Source: CAD feature listing. Evaluate the final solid. Frame: model axes, mm. Give positions to 0.01 mm unless a question says otherwise; leave off trailing zeros. Order: outer loops, then holes, each group sorted by start corner. A loop starts at its lowest first (then second) coordinate and runs counter-clockwise, first axis right, second up. Notation, with made-up numbers: M 9,-3 L 56,-3 A23 ccw 56,34 Z; hole C 45.25,24.25 d11. An arc over 180 degrees is marked long. Answer in a Markdown table with one row per item. Add a question column.
(1) Section query A-A, the plane y = 3.75. Return loops of the section in (x, z) (3 decimals).
(2) Section query B-B, the plane x = 0. Return loops of the section in (y, z) (3 decimals).
(3) Material intervals for line 1 along Z through (x, y) = (0, -11.05); line 2 along Y through (x, z) = (-5.5, 93) (3 decimals); line 3 along X through (y, z) = (10.7, 43.18), sorted ascending.
(4) Pin query (flat end, axial travel): P1, Ø20.5, axis at x = 0, z = 43.18, coming from the +Y side. Return the tip coordinate at first contact, or that it passes through.
(5) Section query C-C, the plane z = 43.18. Return loops of the section in (x, y) (3 decimals), plus the area to 3 significant figures.
(6) Section query D-D, the plane z = 349. Return loops of the section in (x, y) (3 decimals).
from build123d import *

# Parameters (mm, degrees)
SKETCH1_W           = 50.8
SKETCH1_H           = 25.4
SKETCH1_W_2         = 44.45
SKETCH1_H_2         = 19.05
EXTRUDE_THIN1_DEPTH = 508
SKETCH2_R           = 6.35
CUT_EXTRUDE1_DEPTH  = 26.4


with BuildPart() as part:
    # Sketch1 → Extrude-Thin1 (new body)
    with BuildSketch(Plane.XY):
        Rectangle(SKETCH1_W, SKETCH1_H)
        Rectangle(SKETCH1_W_2, SKETCH1_H_2, mode=Mode.SUBTRACT)
    extrude(amount=EXTRUDE_THIN1_DEPTH)

    # Sketch2 → Cut-Extrude1 (cut, through all)
    with BuildSketch(Plane(origin=(0, 12.7, 0), x_dir=(1, 0, 0), z_dir=(0, 1, 0))):
        with Locations((0, -464.82)):
            Circle(SKETCH2_R)
        with Locations((0, -43.18)):
            Circle(SKETCH2_R)
    extrude(amount=-CUT_EXTRUDE1_DEPTH, mode=Mode.SUBTRACT)


solid = part.part
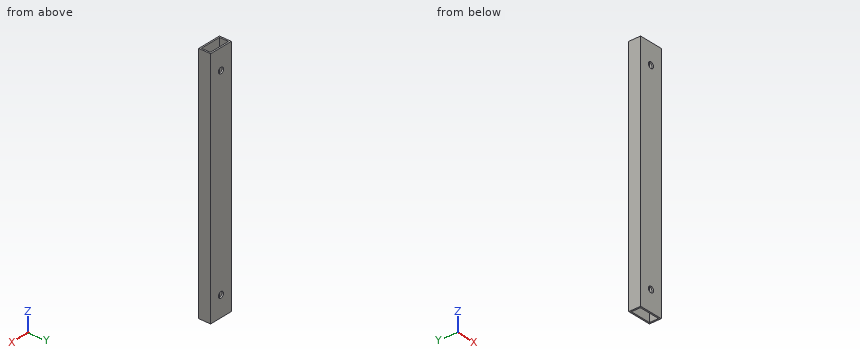
Values follow:
| question | item | result |
|---|---|---|
| 1 | outline | M -25.4,0 L -22.225,0 L -22.225,508 L -25.4,508 Z; M 22.225,0 L 25.4,0 L 25.4,508 L 22.225,508 Z |
| 2 | outline | M -12.7,0 L -9.525,0 L -9.525,36.83 L -12.7,36.83 Z; M -12.7,49.53 L -9.525,49.53 L -9.525,458.47 L -12.7,458.47 Z; M -12.7,471.17 L -9.525,471.17 L -9.525,508 L -12.7,508 Z; M 9.525,0 L 12.7,0 L 12.7,36.83 L 9.525,36.83 Z; M 9.525,49.53 L 12.7,49.53 L 12.7,458.47 L 9.525,458.47 Z; M 9.525,471.17 L 12.7,471.17 L 12.7,508 L 9.525,508 Z |
| 3 | line 1 | z = 0 to 36.83, 49.53 to 458.47, 471.17 to 508 |
| 3 | line 2 | y = -12.7 to -9.525, 9.525 to 12.7 |
| 3 | line 3 | x = -25.4 to -6.35, 6.35 to 25.4 |
| 4 | P1 | stops at y = 12.7 |
| 5 | outline | M -25.4,-12.7 L -6.35,-12.7 L -6.35,-9.525 L -22.225,-9.525 L -22.225,9.525 L -6.35,9.525 L -6.35,12.7 L -25.4,12.7 Z; M 6.35,-12.7 L 25.4,-12.7 L 25.4,12.7 L 6.35,12.7 L 6.35,9.525 L 22.225,9.525 L 22.225,-9.525 L 6.35,-9.525 Z |
| 5 | area | 363 mm² |
| 6 | outline | M -25.4,-12.7 L 25.4,-12.7 L 25.4,12.7 L -25.4,12.7 Z; hole M -22.225,-9.525 L 22.225,-9.525 L 22.225,9.525 L -22.225,9.525 Z |
